Autodesk Inventor part; units mm, degrees
ref_plane "Start Plane" through (0, 0, 0) normal (0, 0, 1) x (1, 0, 0)
ref_plane "End Plane" through (0, 0, 93.0667) normal (0, 0, 1) x (1, 0, 0)
ref_plane "Work Plane4" through (0, 12.7, 0) normal (0.018, 0, -0.9998) x (-0.9998, 0, -0.018)
ref_plane "Start Plane" through (0, 0, 0) normal (0, 0, 1) x (1, 0, 0)
ref_plane "End Plane" through (0, 0, 93.0667) normal (0, 0, 1) x (1, 0, 0)
sketch "Sketch" plane through (0, 0, 0) normal (0, 0, 1) x (1, 0, 0)
  line L0 (25.4, 0) -> (0, 0)
  line L1 (0, 0) -> (0, 25.4)
  line L2 (0, 25.4) -> (1.651, 25.4)
  line L3 (3.175, 23.876) -> (3.175, 6.477)
  line L4 (6.477, 3.175) -> (23.876, 3.175)
  line L5 (25.4, 1.651) -> (25.4, 0)
  line L6 (0, -11.0414) -> (0, 31.5385) construction
  line L7 (-11.0414, 0) -> (31.5385, 0) construction
  arc A0 (3.175, 6.477) -> (6.477, 3.175) centre (6.477, 6.477) ccw
  arc A1 (3.175, 23.876) -> (1.651, 25.4) centre (1.651, 23.876) ccw
  arc A2 (25.4, 1.651) -> (23.876, 3.175) centre (23.876, 1.651) ccw
  line L8 (0, 40.0545) -> (0, -19.5574) construction
  line L9 (-19.5574, 0) -> (40.0545, 0) construction
  point P0 (3.175, 25.4)
  point P1 (3.175, 3.175)
  point P2 (25.4, 3.175)
  dimension "d0" = 25.4
  dimension "d1" = 25.4
  dimension "d2" = 3.175
  dimension "d3" = 3.175
  dimension "d10" = 0
  dimension "d11" = 0
  dimension "d14" = 3.302
  dimension "d15" = 1.524
extrude "Body" add sketch "Sketch" along normal up to surface (93.0667 mm away) from surface at 0
sketch "Sketch3" plane through (0, 0, 0) normal (0, 0, 1) x (1, 0, 0)
  line L0 (0, 0) -> (10, 0)
ref_plane "Work Plane3" through (0, 0, 0) normal (0, -1, 0) x (1, 0, 0)
ref_plane "Work Plane4" through (0, 12.7, 0) normal (0.018, 0, -0.9998) x (-0.9998, 0, -0.018)
split "Split1" plane through (0, 12.7, 0) removes the side toward (0.018, 0, -0.9998)
ref_plane "Work Plane5" through (1.651, 249.7692, 186.5538) normal (0, -0.3846, 0.9231) x (1, 0, 0)
split "Split2" plane through (1.651, 249.7692, 186.5538) removes the side toward (0, -0.3846, 0.9231)
sketch "Sketch4" plane through (0, 0, 0) normal (0, -1, 0) x (1, 0, 0)
  line L0 (-2, 0) -> (12, 0)
  line L1 (-2, 93.0667) -> (12, 93.0667)
  dimension "d17" = 93.0667
equation "\"d0\" = G_H"
equation "\"d1\" = G_H"
equation "\"d2\" = G_T"
equation "\"d3\" = G_T"
equation "\"d14\" = G_IR"
equation "\"d15\" = G_ER"
equation "\"d4\" = G_L"
equation "\"G_H\" = 25.4"
equation "\"G_T\" = 3.175"
equation "\"G_ER\" = 1.524"
equation "\"G_IR\" = 3.302"
equation "\"G_L\" = d17"
equation "\"ex\" = 0"
equation "\"G_OFFSET_START\" = 0"
equation "\"G_OFFSET_END\" = -16.93333"
equation "\"d13\" = G_OFFSET_END + B_L"
equation "\"B_L\" = 110"
properties part number "AISC - L 1 x 1 x 1/8 - 3.664" material "Steel, Mild"
Design review of the part built by this model. Coordinates are the model's own, in mm. A direction names the side the tool comes from. Coordinates: 2 decimals unless noted, no trailing zeros. Order: outer loops, then holes, each group sorted by start corner. A loop starts at its lowest first (then second) coordinate and runs counter-clockwise, first axis right, second up.
Item 1: For pin 1 Ø3 at (x, z) = (15, 39.5) entering from +Y (3 decimals); pin 2 Ø6 at (y, z) = (16.5, 61.5) entering from +X (3 decimals); pin 3 Ø3 at (x, y) = (9.5, 3.5) entering from +Z, all flat-tipped, find the tip position at first contact; note any pin that passes through.
Item 2: Take a section at C-C, the plane y = 19. Write out the cut boundary in (x, z) (3 decimals).
Item 3: Take a section at B-B, the plane x = 16.5. Write out the cut boundary in (y, z) (3 decimals), then the cut area to 3 significant figures.
Item 4: Take a section at D-D, the plane z = 86. Write out the cut boundary in (x, y) (3 decimals), then the cut area to 3 significant figures.
Item 5: Take a section at A-A, the plane z = 31.5. Write out the cut boundary in (x, y) (3 decimals).
Item 6: For line 1 (Y direction, x = 13.5, z = 64) (3 decimals); line 2 (Y direction, x = 1.75, z = 43.5), list the stretches that pass through material, from the lowest coordinate up.
Item 7: For faces 1 (the flat face through (3.175, 15, 46)), 2 (the flat face through (13, 0, 41)), list the 3-axis set-ups (+Z, -Z, +X, -X, +Y, -Y) from which the entire face can be reached by the end or side of a thin tool; tool diameter is ignored.
The answers:
1. pin 1: stops at y = 3.175
1. pin 2: stops at x = 3.175
1. pin 3: stops at z = 83.81
2. outline: (0, 0) - (3.175, 0.057) - (3.175, 90.406) - (0, 90.406) - close
3. outline: (0, 0.297) - (3.175, 0.297) - (3.175, 83.813) - (0, 82.49) - close
3. area: 263 mm2
4. outline: (0, 8.424) - (3.175, 8.424) - (3.175, 23.876) arc R1.524 ccw to (1.651, 25.4) - (0, 25.4) - close
4. area: 53.4 mm2
5. outline: (0, 0) - (25.4, 0) - (25.4, 1.651) arc R1.524 ccw to (23.876, 3.175) - (6.477, 3.175) arc R3.302 cw to (3.175, 6.477) - (3.175, 23.876) arc R1.524 ccw to (1.651, 25.4) - (0, 25.4) - close
6. line 1: y = 0 to 3.175
6. line 2: y = 0 to 25.4
7. face 1: +Z, -Z, +X, +Y
7. face 2: +Z, -Z, +X, -X, -Y
